from build123d import *

# Parameters (mm, degrees)
SKETCH1_R                 = 7.874
BOSS_EXTRUDE1_DEPTH       = 6.35
CUT_EXTRUDE1_REACH        = 8.35
SKETCH2_R                 = 3.175
CUT_EXTRUDE6_REACH        = 8.35
SKETCH8_R                 = 3.127
F_4_CLEARANCE_HOLE1_D     = 2.9464
F_4_CLEARANCE_HOLE1_DEPTH = 6.35
F_4_CLEARANCE_HOLE2_D     = 3.8862
F_4_CLEARANCE_HOLE2_DEPTH = 6.35
CUT_EXTRUDE7_REACH        = 8.35
SKETCH13_R                = 0.79375
CUT_EXTRUDE8_REACH        = 8.35
SKETCH14_R                = 2.38125
F_2_CLEARANCE_HOLE1_D     = 2.9972
F_2_CLEARANCE_HOLE1_DEPTH = 6.35


with BuildPart() as part:
    # Sketch1 → Boss-Extrude1 (new body)
    with BuildSketch(Plane.XY):
        with BuildLine():
            Line((152.4, 69.85), (152.4, -69.85))
            Line((152.4, -69.85), (0, -69.85))
            ThreePointArc((0, -69.85), (-69.85, 0), (0, 69.85))
            Line((0, 69.85), (152.4, 69.85))
        make_face()
        with Locations((69.054102373, -28.60314574)):
            Circle(SKETCH1_R, mode=Mode.SUBTRACT)
        Circle(SKETCH1_R, mode=Mode.SUBTRACT)
    extrude(amount=BOSS_EXTRUDE1_DEPTH)

    # Sketch2 → Cut-Extrude1 (cut, up to next)
    with BuildSketch(Plane.XY.offset(6.35), mode=Mode.PRIVATE) as cut_extrude1_sk1:
        with Locations((76.2, 45.72)):
            Circle(SKETCH2_R)
    cut_extrude1_tool1 = extrude(cut_extrude1_sk1.sketch, amount=-CUT_EXTRUDE1_REACH, mode=Mode.PRIVATE) & part.part
    add(cut_extrude1_tool1.solids().sort_by_distance((76.2, 45.72, 6.35))[0], mode=Mode.SUBTRACT)
    # Sketch2 → Cut-Extrude1 (cut, up to next)
    with BuildSketch(Plane.XY.offset(6.35), mode=Mode.PRIVATE) as cut_extrude1_sk2:
        with Locations((139.7, 45.72)):
            Circle(SKETCH2_R)
    cut_extrude1_tool2 = extrude(cut_extrude1_sk2.sketch, amount=-CUT_EXTRUDE1_REACH, mode=Mode.PRIVATE) & part.part
    add(cut_extrude1_tool2.solids().sort_by_distance((139.7, 45.72, 6.35))[0], mode=Mode.SUBTRACT)

    # Sketch8 → Cut-Extrude6 (cut, up to next)
    with BuildSketch(Plane.XY.offset(6.35), mode=Mode.PRIVATE) as cut_extrude6_sk1:
        with Locations((110.206805808, -4.843621334)):
            Circle(SKETCH8_R)
    cut_extrude6_tool1 = extrude(cut_extrude6_sk1.sketch, amount=-CUT_EXTRUDE6_REACH, mode=Mode.PRIVATE) & part.part
    add(cut_extrude6_tool1.solids().sort_by_distance((110.206806, -4.843621, 6.35))[0], mode=Mode.SUBTRACT)

    # #4 Clearance Hole1
    with Locations(Plane.XY.offset(6.35)):
        with Locations((52.65432584, 53.975), (52.65432584, -53.975)):
            Hole(F_4_CLEARANCE_HOLE1_D / 2, depth=F_4_CLEARANCE_HOLE1_DEPTH)

    # #4 Clearance Hole2
    with Locations(Plane.XY.offset(6.35)):
        with Locations((129.54, 18.415), (147.32, 18.415), (147.32, -4.445), (129.54, -4.445), (138.43, -9.525), (86.36, -14.605), (86.36, -42.545), (137.16, -57.785), (5.073244581, -45.872975683), (-5.061355419, -45.872975683)):
            Hole(F_4_CLEARANCE_HOLE2_D / 2, depth=F_4_CLEARANCE_HOLE2_DEPTH)

    # Sketch13 → Cut-Extrude7 (cut, up to next)
    with BuildSketch(Plane.XY.offset(6.35), mode=Mode.PRIVATE) as cut_extrude7_sk1:
        with Locations((0.005944581, -46.140475683)):
            Circle(SKETCH13_R)
    cut_extrude7_tool1 = extrude(cut_extrude7_sk1.sketch, amount=-CUT_EXTRUDE7_REACH, mode=Mode.PRIVATE) & part.part
    add(cut_extrude7_tool1.solids().sort_by_distance((0.005945, -46.140476, 6.35))[0], mode=Mode.SUBTRACT)

    # Sketch14 → Cut-Extrude8 (cut, up to next)
    with BuildSketch(Plane.XY.offset(6.35), mode=Mode.PRIVATE) as cut_extrude8_sk1:
        with Locations((59.00432584, -53.975)):
            Circle(SKETCH14_R)
    cut_extrude8_tool1 = extrude(cut_extrude8_sk1.sketch, amount=-CUT_EXTRUDE8_REACH, mode=Mode.PRIVATE) & part.part
    add(cut_extrude8_tool1.solids().sort_by_distance((59.004326, -53.975, 6.35))[0], mode=Mode.SUBTRACT)

    # #2 Clearance Hole1
    with Locations(Plane.XY.offset(6.35)):
        with Locations((98.552, 16.383), (124.968, 16.383)):
            Hole(F_2_CLEARANCE_HOLE1_D / 2, depth=F_2_CLEARANCE_HOLE1_DEPTH)


solid = part.part
Build history of the part. All positions in model axes, mm. Give positions to 0.01 mm unless a question says otherwise; leave off trailing zeros. Order: outer loops, then holes, each group sorted by start corner. A loop starts at its lowest first (then second) coordinate and runs counter-clockwise, first axis right, second up. Notation, with made-up numbers: M 89.5,49.5 L 96.5,49.5 A21 cw 96.5,79.5 Z; hole C 77.25,13.25 d2. An arc over 180 degrees is marked long. Put each result on its own line as item: value.
Item 1: Slice it at B-B, the plane z = 3.5. Give the number of separate pieces and of enclosed holes in the cut face, plus the area to 3 significant figures.
From the geometry:
separate pieces: 1
enclosed holes: 21
area: 28,300 mm2
Item 2: Slice it at A-A, the plane x = 66. Write the cut outline in (y, z).
From the geometry:
outline: M -69.85,0 L -35.86,0 L -35.86,6.35 L -69.85,6.35 Z; M -21.35,0 L 69.85,0 L 69.85,6.35 L -21.35,6.35 Z
Item 3: Slice it at C-C, the plane y = 28.5. Write the cut outline in (x, z), plus the area to 3 significant figures.
From the geometry:
outline: M -63.77,0 L 152.4,0 L 152.4,6.35 L -63.77,6.35 Z
area: 1,370 mm2
Item 4: Two-plate mould, pull along X, no slides. Class faces 1 (the cylindrical face through (-69.833, -1.536, 3.131)), 2 (the cylindrical face through (77.9, 48.4, 3.2)), 3 (the flat face through (43, 1, 0)): +X half, -X half, draft (parallel to the pull), parting line (faces both ways), or undercut.
From the geometry:
face 1: -X half
face 2: undercut
face 3: draft
Item 5: Slice it at D-D, the plane x = -43. Write the cut outline in (y, z).
From the geometry:
outline: M -55.05,0 L 55.05,0 L 55.05,6.35 L -55.05,6.35 Z
Item 6: Probe line 1 (Y direction, x = 0, z = 4); line 2 (Y direction, x = 147.32, z = 2); line 3 (X direction, y = 19, z = 4.25). List the from-to ranges inside material, lowest first. Write a range as [from, to].
From the geometry:
line 1: y = [-69.85, -46.93], [-45.35, -7.87], [7.87, 69.85]
line 2: y = [-69.85, -6.39], [-2.5, 16.47], [20.36, 69.85]
line 3: x = [-67.22, 127.69], [131.39, 145.47], [149.17, 152.4]
